Build history of the part. All positions in model axes, mm. Give positions to 0.01 mm unless a question says otherwise; leave off trailing zeros. Order: outer loops, then holes, each group sorted by start corner. A loop starts at its lowest first (then second) coordinate and runs counter-clockwise, first axis right, second up. Notation, with made-up numbers: M 30,87.5 L 41,87.5 A25 cw 41,119.5 Z; hole C 50,-25.5 d3. An arc over 180 degrees is marked long. One line per item, written item: value.
Autodesk Inventor part; units mm, degrees
ref_plane "YZ Plane" through (0, 0, 0) normal (1, 0, 0) x (0, 1, 0)
ref_plane "XZ Plane" through (0, 0, 0) normal (0, 1, 0) x (-1, 0, 0)
ref_plane "XY Plane" through (0, 0, 0) normal (0, 0, 1) x (1, 0, 0)
sketch "Sketch1" plane through (0, 0, 0) normal (1, 0, 0) x (0, 1, 0)
  line L0 (183, 100) -> (-183, 100)
  line L1 (-183, 100) -> (-183, -100)
  line L2 (-183, -100) -> (183, -100)
  line L3 (183, -100) -> (183, 100)
  line L4 (183, 100) -> (-183, -100) construction
  line L5 (-183, 100) -> (183, -100) construction
  point P0 (0, 0)
  dimension "d0" = 366
  dimension "d1" = 200
extrude "Extrusion1" add sketch "Sketch1" along normal blind 3
sketch "Sketch7" plane through (3, 0, 0) normal (1, 0, 0) x (0, 0, -1)
  line L0 (1.5, 50) -> (-1.5, 50)
  line L1 (-1.5, 50) -> (-1.5, -50)
  line L2 (-1.5, -50) -> (1.5, -50)
  line L3 (1.5, -50) -> (1.5, 50)
  line L4 (1.5, 50) -> (-1.5, -50) construction
  line L5 (-1.5, 50) -> (1.5, -50) construction
  point P0 (0, 0)
  dimension "d69" = 3
  dimension "d70" = 100
extrude "Extrusion10" add sketch "Sketch7" along normal blind 24
sketch "Sketch8" plane through (3, -50, 1.5) normal (0, 0, 1) x (1, 0, 0)
  circle A0 centre (13, 75) radius 1.5
  circle A1 centre (13, 50) radius 1.5
  circle A2 centre (13, 25) radius 1.5
  line L0 (0, 100) -> (24, 100)
  line L1 (0, 0) -> (24, 0)
  line L2 (24, 100) -> (24, 0)
  line L3 (0, 233) -> (0, -133)
  point P0 (-3, 50)
  dimension "d73" = 3
  dimension "d74" = 3
  dimension "d75" = 3
  dimension "d76" = 25
  dimension "d77" = 25
  dimension "d78" = 25
  dimension "d87" = 25
  dimension "d88" = 11
  dimension "d89" = 11
  dimension "d90" = 11
extrude "Extrusion11" cut sketch "Sketch8" against normal blind 25 contours A0 | A1 | A2
properties part number "down_cover"
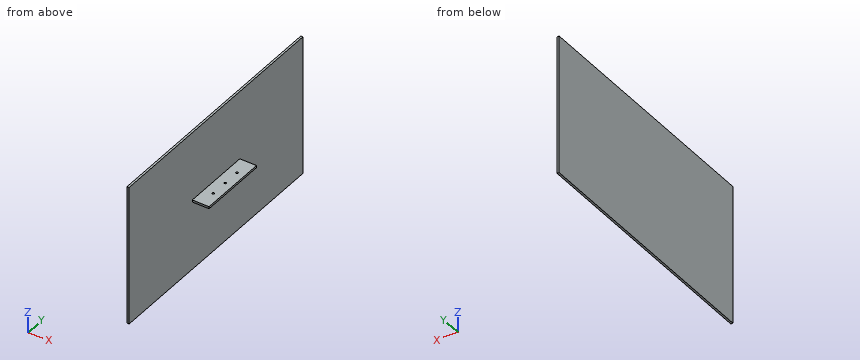
1) Pin check, flat tips, straight feed: pin 1 (1 mm diameter, centred on y = 61.5, z = -41, fed in from +X); pin 2 (7 mm diameter, centred on x = 12, y = -13, fed in from +Z); pin 3 (8 mm diameter, centred on y = 116, z = -77.5, fed in from -X); pin 4 (3.5 mm diameter, centred on x = 14.5, z = 0.5, fed in from +Y). Stop position of each tip, or through.
Check values:
pin 1: x = 3
pin 2: z = 1.5
pin 3: x = 0
pin 4: y = 50
2) Saw through at B-B, the plane y = -56. Write the cut outline in (x, z), then the cut area to 3 significant figures.
Check values:
outline: M 0,-100 L 3,-100 L 3,100 L 0,100 Z
area: 600 mm^2
3) Saw through at A-A, the plane z = -76.5. Write the cut outline in (x, y).
Check values:
outline: M 0,-183 L 3,-183 L 3,183 L 0,183 Z
4) Drill centre lines: probe 1 along Y at (x, z) = (16, 0.05); probe 2 along Z at (x, y) = (21, -32); probe 3 along X at (y, z) = (146.5, -91). Where is each one in solid material? Low to high. Write a range as from..to.
Check values:
probe 1: -50..-26.5, -23.5..-1.5, 1.5..23.5, 26.5..50
probe 2: -1.5..1.5
probe 3: 0..3
